Build history of the part. All positions in model axes, mm. Face numbers are marked on the shaded views. A direction names the side the tool comes from. Round coordinates to 2 decimals unless told otherwise and drop trailing zeros. Loops run counter-clockwise (first coordinate to the right, second up) from the corner with the lowest first, then second, coordinate; pieces in that order, holes last. Notation, with made-up numbers: (-0.75, 65) - (45.25, 65) arc R27 cw to (45.25, 81) - close; hole circle Ø4 at (5.5, 0.25). An arc over 180 degrees is marked (long way). Put each result on its own line as item: value. Start each with the question number.
from build123d import *

# Parameters (mm, degrees)
SKETCH1_W           = 113.8
SKETCH1_H           = 214.8
BOSS_EXTRUDE1_DEPTH = 49.5
SKETCH2_W           = 109.8
SKETCH2_H           = 18.5
CUT_EXTRUDE1_DEPTH  = 42
SKETCH3_W           = 87
SKETCH3_H           = 17.5
BOSS_EXTRUDE2_DEPTH = 7
SKETCH4_W           = 1.5
SKETCH4_H           = 17.5
BOSS_EXTRUDE3_DEPTH = 9.05
SKETCH4_3_W         = 1.5
SKETCH4_3_H         = 17.5
BOSS_EXTRUDE4_DEPTH = 5
SKETCH5_R           = 7
BOSS_EXTRUDE5_DEPTH = 17
SKETCH6_R           = 1.5
CUT_EXTRUDE2_DEPTH  = 5


with BuildPart() as part:
    # Sketch1 → Boss-Extrude1 (new body)
    with BuildSketch(Plane(origin=(0, 0, 0), x_dir=(1, 0, 0), z_dir=(0, 1, 0))):
        Rectangle(SKETCH1_W, SKETCH1_H)
    extrude(amount=BOSS_EXTRUDE1_DEPTH)

    # Sketch2 → Cut-Extrude1 (cut)
    with BuildSketch(Plane(origin=(0, 49.5, 0), x_dir=(1, 0, 0), z_dir=(0, 1, 0))):
        with Locations((0, -98.15)):
            Rectangle(SKETCH2_W, SKETCH2_H)
    extrude(amount=-CUT_EXTRUDE1_DEPTH, mode=Mode.SUBTRACT)

    # Sketch3 → Boss-Extrude2 (add)
    with BuildSketch(Plane(origin=(0, 7.5, 0), x_dir=(1, 0, 0), z_dir=(0, 1, 0))):
        with Locations((7.4, -97.65)):
            Rectangle(SKETCH3_W, SKETCH3_H)
    extrude(amount=BOSS_EXTRUDE2_DEPTH)

    # Sketch4 → Boss-Extrude3 (add)
    with BuildSketch(Plane(origin=(0, 14.5, 0), x_dir=(1, 0, 0), z_dir=(0, 1, 0))):
        with Locations((-35.35, -97.65)):
            Rectangle(SKETCH4_W, SKETCH4_H)
        with Locations((50.15, -97.65)):
            Rectangle(SKETCH4_W, SKETCH4_H)
    extrude(amount=BOSS_EXTRUDE3_DEPTH)

    # Sketch4<3> → Boss-Extrude4 (add)
    with BuildSketch(Plane(origin=(0, 14.5, 0), x_dir=(1, 0, 0), z_dir=(0, 1, 0))):
        with Locations((-25.85, -97.65)):
            Rectangle(SKETCH4_3_W, SKETCH4_3_H)
        with Locations((-16.35, -97.65)):
            Rectangle(SKETCH4_3_W, SKETCH4_3_H)
        with Locations((-6.85, -97.65)):
            Rectangle(SKETCH4_3_W, SKETCH4_3_H)
        with Locations((2.65, -97.65)):
            Rectangle(SKETCH4_3_W, SKETCH4_3_H)
        with Locations((12.15, -97.65)):
            Rectangle(SKETCH4_3_W, SKETCH4_3_H)
        with Locations((21.65, -97.65)):
            Rectangle(SKETCH4_3_W, SKETCH4_3_H)
        with Locations((31.15, -97.65)):
            Rectangle(SKETCH4_3_W, SKETCH4_3_H)
        with Locations((40.65, -97.65)):
            Rectangle(SKETCH4_3_W, SKETCH4_3_H)
    extrude(amount=BOSS_EXTRUDE4_DEPTH)

    # Sketch5 → Boss-Extrude5 (add)
    with BuildSketch(Plane.XY.offset(88.9)):
        with Locations((-43.9, 38)):
            Circle(SKETCH5_R)
    extrude(amount=BOSS_EXTRUDE5_DEPTH)

    # Sketch6 → Cut-Extrude2 (cut)
    with BuildSketch(Plane(origin=(0, 0, 0), x_dir=(-1, 0, 0), z_dir=(0, -1, 0))):
        with Locations((-47.8, -80.6)):
            Circle(SKETCH6_R)
        with Locations((-47.8, 97.4)):
            Circle(SKETCH6_R)
        with Locations((47.4, 97.4)):
            Circle(SKETCH6_R)
        with Locations((47.4, -80.6)):
            Circle(SKETCH6_R)
    extrude(amount=-CUT_EXTRUDE2_DEPTH, mode=Mode.SUBTRACT)


solid = part.part
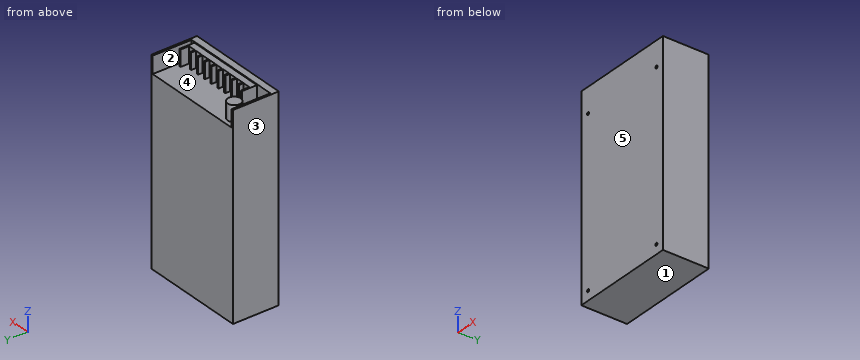
Item 1: Which spindle directions (+Z, -Z, +X, -X, +Y, -Y) get a long thin tool onto all of the face, cutting with end or side? Do the marked faces 1 and 2. Say none if no direction does.
Item 2: Slice it at B-B (x = 35). Give the cut face in (y, z), plus the area to 3 significant figures.
Item 3: Slice it at A-A (y = 38). Give the cut face in (x, z).
Item 4: Two-plate mould, pull along X, no slides. Class the marked faces 3, 4 and 5: pulls with the +X half, pulls with the -X half, needs draft (parallel to the pull), parting line crosses it, or undercut.
Item 5: Drop a flat-ended pin along its axis: pin 1 Ø2.5 at (x, z) = (35, 99.5) entering from +Y. Give the stop position or say it passes through.
Item 6: Drill centre lines: probe 1 along Z at (x, y) = (47.8, 3.2); probe 2 along X at (y, z) = (3, -97.4); probe 3 along X at (y, z) = (3, 80). Where is each one in solid material? Low to high. Write a range as [from, to].
Item 7: Slice it at C-C (x = -43.9). Give the cut face in (y, z), plus the area to 3 significant figures.
Computed values:
1. face 1: -Z, +X, -X, +Y, -Y
1. face 2: +Z, +Y
2. outline: (0, -107.4) - (49.5, -107.4) - (49.5, 88.9) - (14.5, 88.9) - (14.5, 106.4) - (7.5, 106.4) - (7.5, 107.4) - (0, 107.4) - close
2. area: 9,980 mm^2
3. outline: (-56.9, -107.4) - (56.9, -107.4) - (56.9, 107.4) - (54.9, 107.4) - (54.9, 88.9) - (-36.9, 88.9) - (-36.9, 105.9) - (-50.9, 105.9) - (-50.9, 88.9) - (-54.9, 88.9) - (-54.9, 107.4) - (-56.9, 107.4) - close
4. face 3: pulls with the -X half
4. face 4: undercut
4. face 5: needs draft
5. pin 1: stops at y = 14.5
6. probe 1: z = [-107.4, -98.9], [-95.9, 79.1], [82.1, 107.4]
6. probe 2: x = [-56.9, -48.9], [-45.9, 46.3], [49.3, 56.9]
6. probe 3: x = [-56.9, -48.77], [-46.03, 46.43], [49.17, 56.9]
7. outline: (0, -107.4) - (49.5, -107.4) - (49.5, 88.9) - (45, 88.9) - (45, 105.9) - (31, 105.9) - (31, 88.9) - (7.5, 88.9) - (7.5, 107.4) - (0, 107.4) - close
7. area: 10,100 mm^2
